```python
from build123d import *

# Parameters (mm, degrees)
SKETCH1_W           = 200
SKETCH1_H           = 90
BOSS_EXTRUDE1_DEPTH = 6
CUT_EXTRUDE1_REACH  = 111.823
SKETCH2_R           = 16
CUT_EXTRUDE2_REACH  = 111.823
SKETCH3_R           = 3.25
SKETCH3_W           = 12
SKETCH3_H           = 6
SKETCH3_W_2         = 6
SKETCH3_H_2         = 15


with BuildPart() as part:
    # Sketch1 → Boss-Extrude1 (new body)
    with BuildSketch(Plane(origin=(0, 0, 0), x_dir=(1, 0, 0), z_dir=(0, 1, 0))):
        Rectangle(SKETCH1_W, SKETCH1_H)
    extrude(amount=BOSS_EXTRUDE1_DEPTH)

    # Sketch2 → Cut-Extrude1 (cut, up to next)
    with BuildSketch(Plane(origin=(0, 6, 0), x_dir=(1, 0, 0), z_dir=(0, 1, 0)), mode=Mode.PRIVATE) as cut_extrude1_sk1:
        with Locations(Location((-50, 0, 0), (0, 0, 270))):
            Circle(SKETCH2_R)
    cut_extrude1_tool1 = extrude(cut_extrude1_sk1.sketch, amount=-CUT_EXTRUDE1_REACH, mode=Mode.PRIVATE) & part.part
    # Sketch2 → Cut-Extrude1 (cut, up to next)
    with BuildSketch(Plane(origin=(0, 6, 0), x_dir=(1, 0, 0), z_dir=(0, 1, 0)), mode=Mode.PRIVATE) as cut_extrude1_sk2:
        with Locations(Location((50, 0, 0), (0, 0, 270))):
            Circle(SKETCH2_R)
    cut_extrude1_tool2 = extrude(cut_extrude1_sk2.sketch, amount=-CUT_EXTRUDE1_REACH, mode=Mode.PRIVATE) & part.part
    add(cut_extrude1_tool1.solids().sort_by_distance((-50, 6, 0))[0], mode=Mode.SUBTRACT)
    add(cut_extrude1_tool2.solids().sort_by_distance((50, 6, 0))[0], mode=Mode.SUBTRACT)

    # Sketch3 → Cut-Extrude2 (cut, up to next)
    with BuildSketch(Plane(origin=(0, 6, 0), x_dir=(1, 0, 0), z_dir=(0, 1, 0)), mode=Mode.PRIVATE) as cut_extrude2_sk1:
        with Locations(Location((-50, 39, 0), (0, 0, 270))):
            Circle(SKETCH3_R)
    cut_extrude2_tool1 = extrude(cut_extrude2_sk1.sketch, amount=-CUT_EXTRUDE2_REACH, mode=Mode.PRIVATE) & part.part
    # Sketch3 → Cut-Extrude2 (cut, up to next)
    with BuildSketch(Plane(origin=(0, 6, 0), x_dir=(1, 0, 0), z_dir=(0, 1, 0)), mode=Mode.PRIVATE) as cut_extrude2_sk2:
        with Locations(Location((50, 39, 0), (0, 0, 270))):
            Circle(SKETCH3_R)
    cut_extrude2_tool2 = extrude(cut_extrude2_sk2.sketch, amount=-CUT_EXTRUDE2_REACH, mode=Mode.PRIVATE) & part.part
    # Sketch3 → Cut-Extrude2 (cut, up to next)
    with BuildSketch(Plane(origin=(0, 6, 0), x_dir=(1, 0, 0), z_dir=(0, 1, 0)), mode=Mode.PRIVATE) as cut_extrude2_sk3:
        with Locations(Location((50, -39, 0), (0, 0, 270))):
            Circle(SKETCH3_R)
    cut_extrude2_tool3 = extrude(cut_extrude2_sk3.sketch, amount=-CUT_EXTRUDE2_REACH, mode=Mode.PRIVATE) & part.part
    # Sketch3 → Cut-Extrude2 (cut, up to next)
    with BuildSketch(Plane(origin=(0, 6, 0), x_dir=(1, 0, 0), z_dir=(0, 1, 0)), mode=Mode.PRIVATE) as cut_extrude2_sk4:
        with Locations(Location((-50, -39, 0), (0, 0, 270))):
            Circle(SKETCH3_R)
    cut_extrude2_tool4 = extrude(cut_extrude2_sk4.sketch, amount=-CUT_EXTRUDE2_REACH, mode=Mode.PRIVATE) & part.part
    # Sketch3 → Cut-Extrude2 (cut, up to next)
    with BuildSketch(Plane(origin=(0, 6, 0), x_dir=(1, 0, 0), z_dir=(0, 1, 0)), mode=Mode.PRIVATE) as cut_extrude2_sk5:
        with Locations(Location((-94, 0, 0), (0, 0, 270))):
            Circle(SKETCH3_R)
    cut_extrude2_tool5 = extrude(cut_extrude2_sk5.sketch, amount=-CUT_EXTRUDE2_REACH, mode=Mode.PRIVATE) & part.part
    # Sketch3 → Cut-Extrude2 (cut, up to next)
    with BuildSketch(Plane(origin=(0, 6, 0), x_dir=(1, 0, 0), z_dir=(0, 1, 0)), mode=Mode.PRIVATE) as cut_extrude2_sk6:
        with Locations(Location((94, 0, 0), (0, 0, 270))):
            Circle(SKETCH3_R)
    cut_extrude2_tool6 = extrude(cut_extrude2_sk6.sketch, amount=-CUT_EXTRUDE2_REACH, mode=Mode.PRIVATE) & part.part
    # Sketch3 → Cut-Extrude2 (cut, up to next)
    with BuildSketch(Plane(origin=(0, 6, 0), x_dir=(1, 0, 0), z_dir=(0, 1, 0)), mode=Mode.PRIVATE) as cut_extrude2_sk7:
        with Locations((-80, 39)):
            Rectangle(SKETCH3_W, SKETCH3_H)
    cut_extrude2_tool7 = extrude(cut_extrude2_sk7.sketch, amount=-CUT_EXTRUDE2_REACH, mode=Mode.PRIVATE) & part.part
    # Sketch3 → Cut-Extrude2 (cut, up to next)
    with BuildSketch(Plane(origin=(0, 6, 0), x_dir=(1, 0, 0), z_dir=(0, 1, 0)), mode=Mode.PRIVATE) as cut_extrude2_sk8:
        with Locations((-20, 39)):
            Rectangle(SKETCH3_W, SKETCH3_H)
    cut_extrude2_tool8 = extrude(cut_extrude2_sk8.sketch, amount=-CUT_EXTRUDE2_REACH, mode=Mode.PRIVATE) & part.part
    # Sketch3 → Cut-Extrude2 (cut, up to next)
    with BuildSketch(Plane(origin=(0, 6, 0), x_dir=(1, 0, 0), z_dir=(0, 1, 0)), mode=Mode.PRIVATE) as cut_extrude2_sk9:
        with Locations((20, 39)):
            Rectangle(SKETCH3_W, SKETCH3_H)
    cut_extrude2_tool9 = extrude(cut_extrude2_sk9.sketch, amount=-CUT_EXTRUDE2_REACH, mode=Mode.PRIVATE) & part.part
    # Sketch3 → Cut-Extrude2 (cut, up to next)
    with BuildSketch(Plane(origin=(0, 6, 0), x_dir=(1, 0, 0), z_dir=(0, 1, 0)), mode=Mode.PRIVATE) as cut_extrude2_sk10:
        with Locations((80, 39)):
            Rectangle(SKETCH3_W, SKETCH3_H)
    cut_extrude2_tool10 = extrude(cut_extrude2_sk10.sketch, amount=-CUT_EXTRUDE2_REACH, mode=Mode.PRIVATE) & part.part
    # Sketch3 → Cut-Extrude2 (cut, up to next)
    with BuildSketch(Plane(origin=(0, 6, 0), x_dir=(1, 0, 0), z_dir=(0, 1, 0)), mode=Mode.PRIVATE) as cut_extrude2_sk11:
        with Locations((80, -39)):
            Rectangle(SKETCH3_W, SKETCH3_H)
    cut_extrude2_tool11 = extrude(cut_extrude2_sk11.sketch, amount=-CUT_EXTRUDE2_REACH, mode=Mode.PRIVATE) & part.part
    # Sketch3 → Cut-Extrude2 (cut, up to next)
    with BuildSketch(Plane(origin=(0, 6, 0), x_dir=(1, 0, 0), z_dir=(0, 1, 0)), mode=Mode.PRIVATE) as cut_extrude2_sk12:
        with Locations((20, -39)):
            Rectangle(SKETCH3_W, SKETCH3_H)
    cut_extrude2_tool12 = extrude(cut_extrude2_sk12.sketch, amount=-CUT_EXTRUDE2_REACH, mode=Mode.PRIVATE) & part.part
    # Sketch3 → Cut-Extrude2 (cut, up to next)
    with BuildSketch(Plane(origin=(0, 6, 0), x_dir=(1, 0, 0), z_dir=(0, 1, 0)), mode=Mode.PRIVATE) as cut_extrude2_sk13:
        with Locations((-20, -39)):
            Rectangle(SKETCH3_W, SKETCH3_H)
    cut_extrude2_tool13 = extrude(cut_extrude2_sk13.sketch, amount=-CUT_EXTRUDE2_REACH, mode=Mode.PRIVATE) & part.part
    # Sketch3 → Cut-Extrude2 (cut, up to next)
    with BuildSketch(Plane(origin=(0, 6, 0), x_dir=(1, 0, 0), z_dir=(0, 1, 0)), mode=Mode.PRIVATE) as cut_extrude2_sk14:
        with Locations((-80, -39)):
            Rectangle(SKETCH3_W, SKETCH3_H)
    cut_extrude2_tool14 = extrude(cut_extrude2_sk14.sketch, amount=-CUT_EXTRUDE2_REACH, mode=Mode.PRIVATE) & part.part
    # Sketch3 → Cut-Extrude2 (cut, up to next)
    with BuildSketch(Plane(origin=(0, 6, 0), x_dir=(1, 0, 0), z_dir=(0, 1, 0)), mode=Mode.PRIVATE) as cut_extrude2_sk15:
        with Locations((-94, 20)):
            Rectangle(SKETCH3_W_2, SKETCH3_H_2)
    cut_extrude2_tool15 = extrude(cut_extrude2_sk15.sketch, amount=-CUT_EXTRUDE2_REACH, mode=Mode.PRIVATE) & part.part
    # Sketch3 → Cut-Extrude2 (cut, up to next)
    with BuildSketch(Plane(origin=(0, 6, 0), x_dir=(1, 0, 0), z_dir=(0, 1, 0)), mode=Mode.PRIVATE) as cut_extrude2_sk16:
        with Locations((-94, -20)):
            Rectangle(SKETCH3_W_2, SKETCH3_H_2)
    cut_extrude2_tool16 = extrude(cut_extrude2_sk16.sketch, amount=-CUT_EXTRUDE2_REACH, mode=Mode.PRIVATE) & part.part
    # Sketch3 → Cut-Extrude2 (cut, up to next)
    with BuildSketch(Plane(origin=(0, 6, 0), x_dir=(1, 0, 0), z_dir=(0, 1, 0)), mode=Mode.PRIVATE) as cut_extrude2_sk17:
        with Locations((94, -20)):
            Rectangle(SKETCH3_W_2, SKETCH3_H_2)
    cut_extrude2_tool17 = extrude(cut_extrude2_sk17.sketch, amount=-CUT_EXTRUDE2_REACH, mode=Mode.PRIVATE) & part.part
    # Sketch3 → Cut-Extrude2 (cut, up to next)
    with BuildSketch(Plane(origin=(0, 6, 0), x_dir=(1, 0, 0), z_dir=(0, 1, 0)), mode=Mode.PRIVATE) as cut_extrude2_sk18:
        with Locations((94, 20)):
            Rectangle(SKETCH3_W_2, SKETCH3_H_2)
    cut_extrude2_tool18 = extrude(cut_extrude2_sk18.sketch, amount=-CUT_EXTRUDE2_REACH, mode=Mode.PRIVATE) & part.part
    add(cut_extrude2_tool1.solids().sort_by_distance((-50, 6, -39))[0], mode=Mode.SUBTRACT)
    add(cut_extrude2_tool2.solids().sort_by_distance((50, 6, -39))[0], mode=Mode.SUBTRACT)
    add(cut_extrude2_tool3.solids().sort_by_distance((50, 6, 39))[0], mode=Mode.SUBTRACT)
    add(cut_extrude2_tool4.solids().sort_by_distance((-50, 6, 39))[0], mode=Mode.SUBTRACT)
    add(cut_extrude2_tool5.solids().sort_by_distance((-94, 6, 0))[0], mode=Mode.SUBTRACT)
    add(cut_extrude2_tool6.solids().sort_by_distance((94, 6, 0))[0], mode=Mode.SUBTRACT)
    add(cut_extrude2_tool7.solids().sort_by_distance((-80, 6, -39))[0], mode=Mode.SUBTRACT)
    add(cut_extrude2_tool8.solids().sort_by_distance((-20, 6, -39))[0], mode=Mode.SUBTRACT)
    add(cut_extrude2_tool9.solids().sort_by_distance((20, 6, -39))[0], mode=Mode.SUBTRACT)
    add(cut_extrude2_tool10.solids().sort_by_distance((80, 6, -39))[0], mode=Mode.SUBTRACT)
    add(cut_extrude2_tool11.solids().sort_by_distance((80, 6, 39))[0], mode=Mode.SUBTRACT)
    add(cut_extrude2_tool12.solids().sort_by_distance((20, 6, 39))[0], mode=Mode.SUBTRACT)
    add(cut_extrude2_tool13.solids().sort_by_distance((-20, 6, 39))[0], mode=Mode.SUBTRACT)
    add(cut_extrude2_tool14.solids().sort_by_distance((-80, 6, 39))[0], mode=Mode.SUBTRACT)
    add(cut_extrude2_tool15.solids().sort_by_distance((-94, 6, -20))[0], mode=Mode.SUBTRACT)
    add(cut_extrude2_tool16.solids().sort_by_distance((-94, 6, 20))[0], mode=Mode.SUBTRACT)
    add(cut_extrude2_tool17.solids().sort_by_distance((94, 6, 20))[0], mode=Mode.SUBTRACT)
    add(cut_extrude2_tool18.solids().sort_by_distance((94, 6, -20))[0], mode=Mode.SUBTRACT)


solid = part.part
```
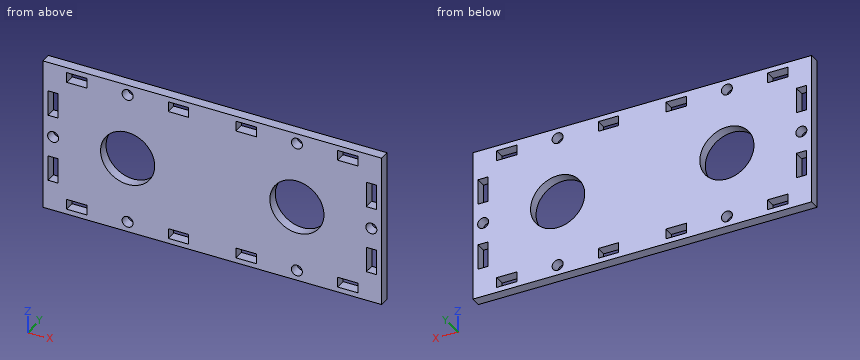
Build history of the part. All positions in model axes, mm. Round coordinates to 2 decimals unless told otherwise and drop trailing zeros. Loops run counter-clockwise (first coordinate to the right, second up) from the corner with the lowest first, then second, coordinate; pieces in that order, holes last. Notation, with made-up numbers: M -7.5,-39.5 L 41.5,-39.5 A22 cw 41.5,-16.5 Z; hole C -25,53 d11. An arc over 180 degrees is marked long. Answer as CSV lines item,"result".
1. Wall check: probe 1 along X at (y, z) = (2.2, -20); probe 2 along Z at (x, y) = (-82, 1); probe 3 along X at (y, z) = (3.3, 0). Give the ranges that are in metal, low to high. Write a range as [from, to].
Resolved:
probe 1,"x = [-100, -97], [-91, 91], [97, 100]"
probe 2,"z = [-45, -42], [-36, 36], [42, 45]"
probe 3,"x = [-100, -97.25], [-90.75, -66], [-34, 34], [66, 90.75], [97.25, 100]"
2. Cut at A-A on z = 0. Write the cut outline in (x, y).
Resolved:
outline,"M -100,0 L -97.25,0 L -97.25,6 L -100,6 Z; M -90.75,0 L -66,0 L -66,6 L -90.75,6 Z; M -34,0 L 34,0 L 34,6 L -34,6 Z; M 66,0 L 90.75,0 L 90.75,6 L 66,6 Z; M 97.25,0 L 100,0 L 100,6 L 97.25,6 Z"
3. Cut at C-C on z = -39. Write the cut outline in (x, y), then the cut area to 3 significant figures.
Resolved:
outline,"M -100,0 L -86,0 L -86,6 L -100,6 Z; M -74,0 L -53.25,0 L -53.25,6 L -74,6 Z; M -46.75,0 L -26,0 L -26,6 L -46.75,6 Z; M -14,0 L 14,0 L 14,6 L -14,6 Z; M 26,0 L 46.75,0 L 46.75,6 L 26,6 Z; M 53.25,0 L 74,0 L 74,6 L 53.25,6 Z; M 86,0 L 100,0 L 100,6 L 86,6 Z"
area,"834 mm²"
4. Cut at B-B on x = -50. Write the cut outline in (y, z), then the cut area to 3 significant figures.
Resolved:
outline,"M 0,-45 L 6,-45 L 6,-42.25 L 0,-42.25 Z; M 0,-35.75 L 6,-35.75 L 6,-16 L 0,-16 Z; M 0,16 L 6,16 L 6,35.75 L 0,35.75 Z; M 0,42.25 L 6,42.25 L 6,45 L 0,45 Z"
area,"270 mm²"
5. Cut at D-D on x = 16. Write the cut outline in (y, z).
Resolved:
outline,"M 0,-45 L 6,-45 L 6,-42 L 0,-42 Z; M 0,-36 L 6,-36 L 6,36 L 0,36 Z; M 0,42 L 6,42 L 6,45 L 0,45 Z"
